from build123d import *

# Parameters (mm, degrees)
SKETCH1_W           = 23
SKETCH1_H           = 47
BOSS_EXTRUDE1_DEPTH = 75
CUT_EXTRUDE1_REACH  = 91.254
FILLET1_R           = 3
FILLET2_R           = 1


with BuildPart() as part:
    # Sketch1 → Boss-Extrude1 (new body)
    with BuildSketch(Plane(origin=(0, 0, 0), x_dir=(1, 0, 0), z_dir=(0, 1, 0))):
        Rectangle(SKETCH1_W, SKETCH1_H)
    extrude(amount=-BOSS_EXTRUDE1_DEPTH)

    # Sketch2 → Cut-Extrude1 (cut, up to next)
    with BuildSketch(Plane.XY.offset(23.5), mode=Mode.PRIVATE) as cut_extrude1_sk1:
        with BuildLine():
            Line((-8.131919427, -61.241229517), (-11.5, -60.015348442))
            Line((-11.5, -60.015348442), (-11.5, -75))
            Line((-11.5, -75), (-5.5, -75))
            Line((-5.5, -75), (-5.5, -65))
            ThreePointArc((-5.5, -65), (-6.223391823, -62.705694255), (-8.131919427, -61.241229517))
        make_face()
    cut_extrude1_tool1 = extrude(cut_extrude1_sk1.sketch, amount=-CUT_EXTRUDE1_REACH, mode=Mode.PRIVATE) & part.part
    add(cut_extrude1_tool1.solids().sort_by_distance((-8.622504, -68.134359, 23.5))[0], mode=Mode.SUBTRACT)

    # Fillet1
    fillet1_edges = [part.edges().sort_by_distance(p)[0] for p in [
        (-5.5, -75, 0),
    ]]
    fillet(fillet1_edges, radius=FILLET1_R)

    # Fillet2
    fillet2_edges = [part.edges().sort_by_distance(p)[0] for p in [
        (11.5, -37.5, 23.5),
        (11.5, -37.5, -23.5),
    ]]
    fillet(fillet2_edges, radius=FILLET2_R)


solid = part.part
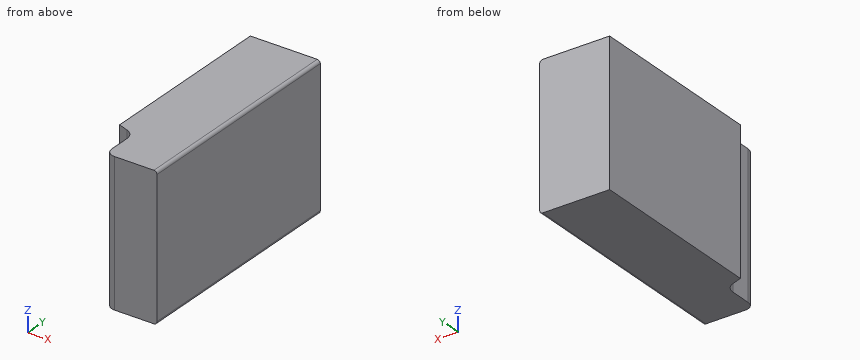
Verification items for the finished model (mm, model axes). Coordinates: 2 decimals unless noted, no trailing zeros. Write each loop counter-clockwise with the first axis right and the second up, starting at its lowest first coordinate (ties: lowest second). Pieces come first, ordered by that corner, then holes. Notation, with made-up numbers: M 36,50 L 70,50 A9 ccw 70,63 Z; hole C 61.25,32 d1. An arc over 180 degrees is marked long. One line per question, with ' | ' between items.
1) Sectioned sample at A-A on z = 20. Record the cut outline in (x, y), then the cut area to 3 significant figures.
Solutions:
outline: M -11.5,-60.02 L -8.13,-61.24 A4 cw -5.5,-65 L -5.5,-72 A3 ccw -2.5,-75 L 11.5,-75 L 11.5,0 L -11.5,0 Z | area: 1,640 mm^2
2) Material ranges on L1, parallel to X at y = -69, z = 19.5; L2, parallel to Y at x = -7, z = 12; L3, parallel to Y at x = -7.25, z = 9, recorded low to high.
Solutions:
L1: -5.5 to 11.5 | L2: -61.88 to 0 | L3: -61.69 to 0
3) Depth check by flat-ended pin: pin 1 Ø5.5 at (y, z) = (-69.5, 3) entering from -X. Enter the tip coordinate at first touch or a pass-through.
Solutions:
pin 1: x = -5.5
4) Sectioned sample at B-B on y = -68. Record the cut outline in (x, z), then the cut area to 3 significant figures.
Solutions:
outline: M -5.5,-23.5 L 10.5,-23.5 A1 ccw 11.5,-22.5 L 11.5,22.5 A1 ccw 10.5,23.5 L -5.5,23.5 Z | area: 799 mm^2
